Geometry: final body of the model. Coordinates: model frame, mm. Face numbers are marked on the shaded views. A direction names the side the tool comes from. Coordinates: 2 decimals unless noted, no trailing zeros. Write each loop counter-clockwise with the first axis right and the second up, starting at its lowest first coordinate (ties: lowest second). Pieces come first, ordered by that corner, then holes. Notation, with made-up numbers: (-13, 39) - (12, 39) arc R37 ccw to (12, 77) - close; hole circle Ø7 at (81, -16.75). An arc over 180 degrees is marked (long way). Answer as a JSON object with one key per item and string values. Group by question number.
Item 1: First-contact query: pin 1 Ø1 at (x, z) = (47, 15.5) entering from -Y; pin 2 Ø4 at (x, z) = (30.5, 4.5) entering from +Y; pin 3 Ø9 at (x, z) = (32, 6) entering from +Y; pin 4 Ø4 at (y, z) = (29.5, 3) entering from -X. Flat tips, straight axial feed; report the tip coordinate or a pass-through.
Item 2: Mould query, pull axis X, two halves, no side actions, for the marked faces 4, 5 and 6. Classes: pulls with the +X half, pulls with the -X half, needs draft (parallel to the pull), parting line crosses it, or undercut.
Item 3: Line query: line 1 along Z through (x, y) = (44.5, 5.25); line 2 along Y through (x, z) = (15.5, 14.25); line 3 along X through (y, z) = (29, 9.75). Output: solid intervals per line, ascending. Write a range as from..to.
Item 4: Section B-B on x = 44.5. Return loops of the section in (y, z).
Item 5: Section A-A on z = 7.25. State how many separate pieces and enclosed holes the cut face has, and give its area (3 significant figures).
Item 6: Section D-D on y = 8.5. Return loops of the section in (x, z), and give its area (3 significant figures).
Item 7: Set-up query: the marked faces 1, 2 and 3. Return all of +Z, -Z, +X, -X, +Y, -Y with unobstructed straight access to the full face (end or side cutting, diameter ignored); none if empty.
Autodesk Inventor part; units mm, degrees
ref_plane "YZ Plane" through (0, 0, 0) normal (1, 0, 0) x (0, 1, 0)
ref_plane "XZ Plane" through (0, 0, 0) normal (0, 1, 0) x (-1, 0, 0)
ref_plane "XY Plane" through (0, 0, 0) normal (0, 0, 1) x (1, 0, 0)
sketch "Sketch1" plane through (0, 0, 0) normal (0, 0, 1) x (1, 0, 0)
  line L0 (0, 0) -> (59, 0)
  line L1 (7, 3) -> (22, 3)
  line L2 (7, 3) -> (22, 3) construction
  line L3 (0, 0) -> (41.7193, 41.7193)
  line L4 (0, 0) -> (59, 0) construction
  line L5 (7, 3) -> (17.6066, 13.6066)
  line L6 (7, 3) -> (22, 3) construction
  line L7 (17.6066, 13.6066) -> (22, 3)
  line L8 (59, 0) -> (59, 6.89)
  line L9 (59, 6.89) -> (24, 6.89)
  line L10 (41.7193, 41.7193) -> (46.5913, 36.8473)
  line L11 (46.5913, 36.8473) -> (21.8425, 12.0986)
  line L12 (21.8425, 12.0986) -> (24.3232, 6.89)
  dimension "d0" = 59
  dimension "d1" = 15
  dimension "d3" = 59
  dimension "d4" = 45
  dimension "d5" = 15
  dimension "d6" = 45
  dimension "d7" = 6.89
  dimension "d8" = 35
  dimension "d10" = 6.89
  dimension "d11" = 35
extrude "Extrusion1" add sketch "Sketch1" along normal blind 18
sketch "Sketch2" plane through (0, 0, 18) normal (0, 0, 1) x (1, 0, 0)
  point P0 (0, 0)
fillet "Fillet1" radius 6.89 1 edges at (46.5913, 36.8473, 9)
fillet "Fillet2" radius 6.89 1 edges at (59, 6.89, 9)
sketch "Sketch3" plane through (24.3232, 6.89, 18) normal (0, 1, 0) x (1, 0, 0)
  point P0 (-24.3232, 18)
sketch "Sketch4" plane through (0, 0, 0) normal (0, -1, 0) x (1, 0, 0)
  point P0 (0, 0)
sketch "Sketch5" plane through (0, 0, 0) normal (0, -1, 0) x (1, 0, 0)
  circle A0 centre (44.5, 9) radius 2.5
  point P0 (0, 0)
  dimension "d16" = 5
extrude "Extrusion2" cut sketch "Sketch5" against normal blind 6.89
sketch "Sketch6" plane through (0, 0, 0) normal (-0.7071, 0.7071, 0) x (-0.7071, -0.7071, 0)
  circle A0 centre (-44.5, 9) radius 2.5
  point P0 (0, 0)
  dimension "d19" = 5
extrude "Extrusion3" cut sketch "Sketch6" against normal blind 6.89
properties part number "45 Degree Connector"
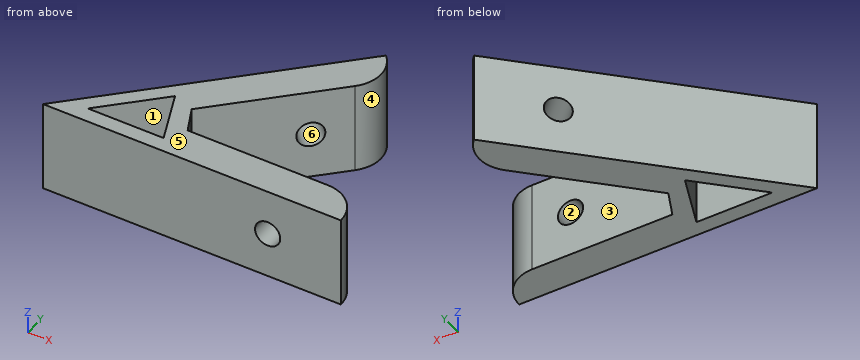
Checks:
{
 "1": {"pin 1": "y = 0", "pin 2": "y = 32.5", "pin 3": "y = 36.5", "pin 4": "x = 27.5"},
 "2": {"face 4": "pulls with the +X half", "face 5": "needs draft", "face 6": "undercut"},
 "3": {"line 1": "0..6.5, 11.5..18", "line 2": "0..3, 11.5..15.5", "line 3": "29..30.56, 37.31..38.74"},
 "4": {"outline": "(0, 0) - (6.89, 0) - (6.89, 6.5) - (0, 6.5) - close; (0, 11.5) - (6.89, 11.5) - (6.89, 18) - (0, 18) - close"},
 "5": {"separate pieces": "3", "enclosed holes": "1", "area": "569 mm^2"},
 "6": {"outline": "(8.5, 0) - (12.5, 0) - (12.5, 18) - (8.5, 18) - close; (19.72, 0) - (23.56, 0) - (23.56, 18) - (19.72, 18) - close", "area": "141 mm^2"},
 "7": {"face 1": "+Z, -Z", "face 2": "-Y", "face 3": "+Z, -Z, +X"}
}
